from build123d import *

# Parameters (mm, degrees)
SKETCH1_R                    = 2.5
BOSS_EXTRUDE1_DEPTH          = 8
SKETCH6_R                    = 0.25
CUT_EXTRUDE1_DEPTH           = 1
CHAMFER1_SIZE                = 2.2
CHAMFER1_SIZE2               = 0.844500877
SKETCH7_W                    = 1.688266385
SKETCH7_H                    = 5.007188161
CUT_EXTRUDE2_DEPTH           = 5
F_2_0_2_DIAMETER_HOLE1_D     = 2
F_2_0_2_DIAMETER_HOLE1_DEPTH = 7.05
F_2_0_2_DIAMETER_HOLE1_TIP   = 0.600860619


with BuildPart() as part:
    # Sketch1 → Boss-Extrude1 (new body)
    with BuildSketch(Plane.XY):
        Circle(SKETCH1_R)
    extrude(amount=BOSS_EXTRUDE1_DEPTH)

    # Sketch6 → Cut-Extrude1 (cut)
    with BuildSketch(Plane(origin=(0, 0, 0), x_dir=(-1, 0, 0), z_dir=(0, 0, -1))):
        Circle(SKETCH6_R)
    extrude(amount=-CUT_EXTRUDE1_DEPTH, mode=Mode.SUBTRACT)

    # Chamfer1
    chamfer1_edges = [part.edges().sort_by_distance(p)[0] for p in [
        (-2.5, 0, 0),
    ]]
    chamfer1_side = [part.faces().sort_by_distance(p)[0] for p in [
        (-2.429289322, 0, 0),
    ]]
    chamfer(chamfer1_edges, length=CHAMFER1_SIZE, length2=CHAMFER1_SIZE2, reference=chamfer1_side[0])

    # Sketch7 → Cut-Extrude2 (cut, symmetric)
    with BuildSketch(Plane(origin=(0, 0, 0), x_dir=(1, 0, 0), z_dir=(0, 1, 0))):
        with Locations((2.594133193, -1.496405919)):
            Rectangle(SKETCH7_W, SKETCH7_H)
    cut_extrude2 = extrude(amount=CUT_EXTRUDE2_DEPTH, both=True, mode=Mode.SUBTRACT)

    # Mirror1: Cut-Extrude2 across plane
    add(cut_extrude2.mirror(Plane(origin=(0, 0, 0), x_dir=(0, 0, 1), z_dir=(1, 0, 0))), mode=Mode.SUBTRACT)

    # Ø2.0 (2) Diameter Hole1
    with Locations(Plane.XY.offset(8)):
        with Locations((0, 0)):
            Hole(F_2_0_2_DIAMETER_HOLE1_D / 2, depth=F_2_0_2_DIAMETER_HOLE1_DEPTH)
            with Locations((0, 0, -(F_2_0_2_DIAMETER_HOLE1_DEPTH + F_2_0_2_DIAMETER_HOLE1_TIP / 2))):  # 118° drill point
                Cone(0, F_2_0_2_DIAMETER_HOLE1_D / 2, F_2_0_2_DIAMETER_HOLE1_TIP, mode=Mode.SUBTRACT)


solid = part.part
Read the model definition and answer for the solid it produces. Units are mm, in the model's axes. A direction names the side the tool comes from. Round coordinates to 2 decimals unless told otherwise and drop trailing zeros. Write each loop counter-clockwise with the first axis right and the second up, starting at its lowest first coordinate (ties: lowest second). Pieces come first, ordered by that corner, then holes. Notation, with made-up numbers: (4.5, 79) - (50.5, 79) arc R34 cw to (50.5, 114) - close; hole circle Ø4 at (-34, 55.5). An arc over 180 degrees is marked (long way). Use a Markdown table: item, result.
(1) Which of the six approach directions +Z, -Z, +X, -X, +Y, -Y give full straight-line access (tool end or side, diameter ignored) to faces 4 (the flat face through (-1.75, 0, 2)), 5 (the flat face through (1.75, 0, 2))?
Reported:
| item | result |
|---|---|
| face 4 | -Z, -X, +Y, -Y |
| face 5 | -Z, +X, +Y, -Y |
(2) The part is cut by section C-C (z = 5). Write down the section's boundary in (x, y), then the cut area to 3 significant figures.
Reported:
| item | result |
|---|---|
| outline | circle Ø5 at (0, 0); hole circle Ø2 at (0, 0) |
| area | 16.5 mm2 |
(3) Straight lines are drawn through the part: line 1 along Y through (x, z) = (0, 6.25); line 2 along X through (y, z) = (0, 3.75); line 3 along Y through (x, z) = (0.85, 3.5). For each, find the intervals that lie inside material, in ascending order. Write a range as [from, to].
Reported:
| item | result |
|---|---|
| line 1 | [-2.5, -1], [1, 2.5] |
| line 2 | [-1.75, -1], [1, 1.75] |
| line 3 | [-2.35, -0.53], [0.53, 2.35] |
(4) Each of these flat-tipped pins is pushed along its axis until it touches: pin 1 Ø1.6 at (x, y) = (0, 0) entering from +Z; pin 2 Ø0.6 at (x, y) = (2, 0.5) entering from -Z; pin 3 Ø1 at (x, y) = (0, 1) entering from -Z. Where does it stop, or does it pass through?
Reported:
| item | result |
|---|---|
| pin 1 | z = 0.83 |
| pin 2 | z = 0.56 |
| pin 3 | z = 0.08 |
(5) The mould has two halves that part along Y. Classify faces 1 (the cylindrical face through (0, -1, 4)), 2 (the cylindrical face through (2.385, 0.751, 5.167)), 3 (the flat face through (1, -1, 8)): released by +Y, released by -Y, zero draft, split by the parting line, or undercut.
Reported:
| item | result |
|---|---|
| face 1 | undercut |
| face 2 | split by the parting line |
| face 3 | zero draft |
(6) The part is cut by section B-B (y = 0). Write down the section's boundary in (x, z).
Reported:
| item | result |
|---|---|
| outline | (-2.5, 4) - (-1.75, 4) - (-1.75, 0.56) - (-0.3, 0) - (-0.25, 0) - (-0.25, 0.5) - (-1, 0.95) - (-1, 8) - (-2.5, 8) - close; (0.25, 0) - (0.3, 0) - (1.75, 0.56) - (1.75, 4) - (2.5, 4) - (2.5, 8) - (1, 8) - (1, 0.95) - (0.25, 0.5) - close |
(7) The part is cut by section A-A (x = 0). Write down the section's boundary in (y, z), then the cut area to 3 significant figures.
Reported:
| item | result |
|---|---|
| outline | (-2.5, 0.84) - (-0.3, 0) - (-0.25, 0) - (-0.25, 0.5) - (-1, 0.95) - (-1, 8) - (-2.5, 8) - close; (0.25, 0) - (0.3, 0) - (2.5, 0.84) - (2.5, 8) - (1, 8) - (1, 0.95) - (0.25, 0.5) - close |
| area | 23.2 mm2 |
